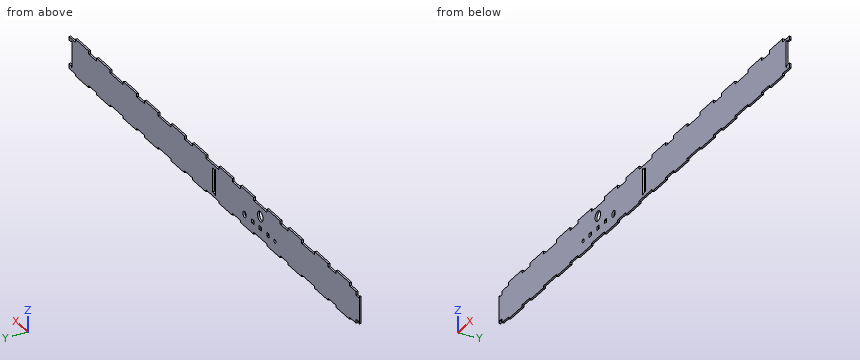
from build123d import *

# Parameters (mm, degrees)
F0_W      = 834.7400754492
F0_H      = 50.8
F1_DEPTH  = 3.048
F3_W      = 57.9247
F3_H      = 5.08
F3_W_2    = 115.8494
F3_H_2    = 3.1496
F4_DEPTH  = 3.048
F6_DEPTH  = 3.048
F7_DEPTH  = 3.049
F9_W      = 6.096
F9_H      = 6.096
F9_R      = 2.8702
F9_R_2    = 4.953
F9_R_3    = 7.9375
F10_DEPTH = 3.049
F11_DEPTH = 25.4
F12_W     = 38.1
F12_H     = 3.048
F12_H_2   = 5.08
F13_DEPTH = 3.048


# Not quite as in the source:
# - a feature names something its author has since deleted; it is built from what else it names


with BuildPart() as f1:
    # F0 (on Front) → F1 (new body)
    with BuildSketch(Plane.XZ):
        with Locations((417.3700377246, 25.4)):
            Rectangle(F0_W, F0_H)
    extrude(amount=F1_DEPTH)

    # F3 (on face) → F4 (join)
    with BuildSketch(Plane.XZ.offset(3.048)):
        with Locations((28.96235, 53.34)):
            Rectangle(F3_W, F3_H)
        with Locations((139.1233459082, 53.34)):
            Rectangle(F3_W_2, F3_H)
        with Locations((278.2466918164, 53.34)):
            Rectangle(F3_W_2, F3_H)
        with Locations((417.3700377246, 53.34)):
            Rectangle(F3_W_2, F3_H)
        with Locations((556.4933836328, 53.34)):
            Rectangle(F3_W_2, F3_H)
        with Locations((695.616729541, 53.34)):
            Rectangle(F3_W_2, F3_H)
        with Locations((805.7777254492, 53.34)):
            Rectangle(F3_W, F3_H)
        with Locations((28.96235, -1.5748)):
            Rectangle(F3_W, F3_H_2)
        with Locations((139.1233459082, -1.5748)):
            Rectangle(F3_W_2, F3_H_2)
        with Locations((278.2466918164, -1.5748)):
            Rectangle(F3_W_2, F3_H_2)
        with Locations((417.3700377246, -1.5748)):
            Rectangle(F3_W_2, F3_H_2)
        with Locations((556.4933836328, -1.5748)):
            Rectangle(F3_W_2, F3_H_2)
        with Locations((695.616729541, -1.5748)):
            Rectangle(F3_W_2, F3_H_2)
        with Locations((805.7777254492, -1.5748)):
            Rectangle(F3_W, F3_H_2)
    extrude(amount=-F4_DEPTH)

    # F5 (on face) → F6 (join)
    with BuildSketch(Plane.XZ.offset(3.048)):
        Polygon((-6.35, 6.35), (0, 6.35), (0, 44.45), (-6.35, 44.45), (-9.525, 47.625), (-9.525, 3.175), align=None)
    extrude(amount=-F6_DEPTH)

    # F5 (on face) → F7 (cut, through all)
    with BuildSketch(Plane.XZ.offset(3.048)):
        Polygon((828.3900754492, 7.3152), (834.7400754492, 7.3152), (834.7400754492, 45.4152), (828.3900754492, 45.4152), (825.2150754492, 48.5902), (825.2150754492, 4.1402), align=None)
    extrude(amount=-F7_DEPTH, mode=Mode.SUBTRACT)

    # F9 (on face) → F10 (cut, through all)
    with BuildSketch(Plane.XZ.offset(3.048)):
        with Locations((256.3264918164, 15.621)):
            Rectangle(F9_W, F9_H)
        with Locations((278.2466918164, 15.621)):
            Rectangle(F9_W, F9_H)
        with Locations((300.1668918164, 15.621)):
            Rectangle(F9_W, F9_H)
        with Locations((235.7016918164, 15.621)):
            Circle(F9_R)
        with Locations((323.9666918164, 15.621)):
            Circle(F9_R_2)
        with Locations((278.2466918164, 34.671)):
            Circle(F9_R_3)
    extrude(amount=-F10_DEPTH, mode=Mode.SUBTRACT)

    # F8 (on face) → F11 (cut)
    with BuildSketch(Plane.XZ.offset(3.048)):
        Polygon((411.0200377246, 6.35), (417.3700377246, 6.35), (417.3700377246, 44.45), (411.0200377246, 44.45), (407.8450377246, 47.625), (407.8450377246, 3.175), align=None)
    extrude(amount=-F11_DEPTH, mode=Mode.SUBTRACT)

    # F12 (on face) → F13 (cut, through all)
    with BuildSketch(Plane.XZ.offset(3.048)):
        with Locations((139.1233459082, -1.6256)):
            Rectangle(F12_W, F12_H)
        with Locations((278.2466918164, -1.6256)):
            Rectangle(F12_W, F12_H)
        with Locations((417.3700377246, -1.6256)):
            Rectangle(F12_W, F12_H)
        with Locations((556.4933836328, -1.6256)):
            Rectangle(F12_W, F12_H)
        with Locations((695.616729541, -1.6256)):
            Rectangle(F12_W, F12_H)
        with Locations((834.7400754492, -1.6256)):
            Rectangle(F12_W, F12_H)
        with Locations((0, -1.6256)):
            Rectangle(F12_W, F12_H)
        with Locations((0, 53.34)):
            Rectangle(F12_W, F12_H_2)
        with Locations((139.1233459082, 53.34)):
            Rectangle(F12_W, F12_H_2)
        with Locations((278.2466918164, 53.34)):
            Rectangle(F12_W, F12_H_2)
        with Locations((417.3700377246, 53.34)):
            Rectangle(F12_W, F12_H_2)
        with Locations((556.4933836328, 53.34)):
            Rectangle(F12_W, F12_H_2)
        with Locations((695.616729541, 53.34)):
            Rectangle(F12_W, F12_H_2)
        with Locations((834.7400754492, 53.34)):
            Rectangle(F12_W, F12_H_2)
    extrude(amount=-F13_DEPTH, mode=Mode.SUBTRACT)


solid = f1.part
The model under review builds one solid part; all positions refer to its coordinate system, in mm. Round coordinates to 2 decimals unless told otherwise and drop trailing zeros. Answer as CSV lines item,"result". Start each with the question number.
Item 1: Consider section A-A (y = -0.9). State how many separate pieces and enclosed holes the cut face has, then the cut area to 3 significant figures.
Item 2: Wall thickness on line 1 (X direction, y = -2.2, z = 31) (3 decimals); line 2 (Z direction, x = 411.5, y = -1.6); line 3 (X direction, y = -2.75, z = 41) (3 decimals): over which ranges is each line inside the solid? List them lowest first. Write a range as [from, to].
Item 3: Insertion check: P1, Ø1.5, axis at y = -1.5, z = -2, coming from the -X side; P2, Ø0.9, axis at y = -2, z = -2, coming from the +X side; P3, Ø1.5, axis at x = 69.5, y = -1, coming from the -Z side. Each pin has a flat end and moves straight along its axis. Give the tip position at first contact, or say it passes through.
Answer:
1,separate pieces,"1"
1,enclosed holes,"7"
1,area,"45,500 mm^2"
2,line 1,"x = [-9.525, 271.209], [285.284, 407.845], [417.37, 825.215]"
2,line 2,"z = [-0.1, 6.35], [44.45, 50.8]"
2,line 3,"x = [-9.525, 273.456], [283.037, 407.845], [417.37, 825.215]"
3,P1,"stops at x = 19.05"
3,P2,"stops at x = 815.69"
3,P3,"stops at z = 0"
